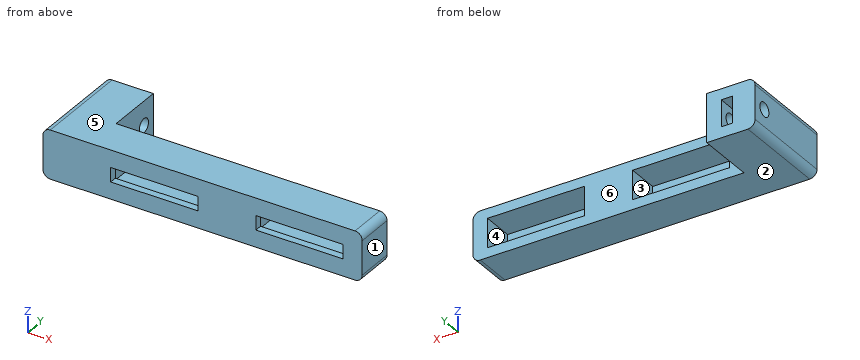
```python
from build123d import *

# Parameters (mm, degrees)
SALIENTE_EXTRUIR1_DEPTH = 10
REDONDEO5_R             = 1.5
CROQUIS3_W              = 20
CROQUIS3_H              = 6
CORTAR_EXTRUIR1_DEPTH   = 6.5
CROQUIS4_W              = 18
CROQUIS4_H              = 2.95
CORTAR_EXTRUIR2_DEPTH   = 1.5
CROQUIS5_R              = 1.45
CORTAR_EXTRUIR3_DEPTH   = 10
CROQUIS6_W              = 2.35
CROQUIS6_H              = 5.5
CORTAR_EXTRUIR4_DEPTH   = 6


with BuildPart() as part:
    # Croquis2 → Saliente-Extruir1 (new body)
    with BuildSketch(Plane.XY):
        Polygon((-160.336548935, 23.55779901), (-160.336548935, 3.55779901), (-94.336548935, 3.55779901), (-94.336548935, 11.55779901), (-150.336548935, 11.55779901), (-150.336548935, 23.55779901), align=None)
    extrude(amount=SALIENTE_EXTRUIR1_DEPTH)

    # Redondeo5
    redondeo5_edges = [part.edges().sort_by_distance(p)[0] for p in [
        (-94.336548935, 7.55779901, 10),
        (-94.336548935, 7.55779901, 0),
        (-160.336548935, 13.55779901, 10),
        (-160.336548935, 13.55779901, 0),
    ]]
    fillet(redondeo5_edges, radius=REDONDEO5_R)

    # Croquis3 → Cortar-Extruir1 (cut)
    with BuildSketch(Plane(origin=(0, 11.55779901, 0), x_dir=(1, 0, 0), z_dir=(0, 1, 0))):
        with Locations((-107.336548935, -5)):
            Rectangle(CROQUIS3_W, CROQUIS3_H)
        with Locations((-137.336548935, -5)):
            Rectangle(CROQUIS3_W, CROQUIS3_H)
    extrude(amount=-CORTAR_EXTRUIR1_DEPTH, mode=Mode.SUBTRACT)

    # Croquis4 → Cortar-Extruir2 (cut)
    with BuildSketch(Plane(origin=(0, 5.05779901, 0), x_dir=(1, 0, 0), z_dir=(0, 1, 0))):
        with Locations((-107.336548935, -4.975)):
            Rectangle(CROQUIS4_W, CROQUIS4_H)
        with Locations((-137.336548935, -4.975)):
            Rectangle(CROQUIS4_W, CROQUIS4_H)
    extrude(amount=-CORTAR_EXTRUIR2_DEPTH, mode=Mode.SUBTRACT)

    # Croquis5 → Cortar-Extruir3 (cut)
    with BuildSketch(Plane(origin=(-150.336548935, 0, 0), x_dir=(0, 0, -1), z_dir=(1, 0, 0))):
        with Locations((-5, 20.55779901)):
            Circle(CROQUIS5_R)
    extrude(amount=-CORTAR_EXTRUIR3_DEPTH, mode=Mode.SUBTRACT)

    # Croquis6 → Cortar-Extruir4 (cut)
    with BuildSketch(Plane(origin=(0, 23.55779901, 0), x_dir=(1, 0, 0), z_dir=(0, 1, 0))):
        with Locations((-154.511548935, -5)):
            Rectangle(CROQUIS6_W, CROQUIS6_H)
    extrude(amount=-CORTAR_EXTRUIR4_DEPTH, mode=Mode.SUBTRACT)


solid = part.part
```
CAD build for the part. Positions are in the model's coordinates, mm. Face numbers are marked on the shaded views. A direction names the side the tool comes from. Round coordinates to 2 decimals unless told otherwise and drop trailing zeros. Order: outer loops, then holes, each group sorted by start corner. A loop starts at its lowest first (then second) coordinate and runs counter-clockwise, first axis right, second up. Notation, with made-up numbers: (11.25, 11.5) - (69.25, 11.5) arc R35 cw to (69.25, 50.5) - close; hole circle Ø1 at (40, 3). An arc over 180 degrees is marked (long way). Answer as CSV lines item,"result". Start each with the question number.
1. Drill centre lines: L1, parallel to X at y = 10.5, z = 4.5; L2, parallel to Z at x = -134.5, y = 5.5; L3, parallel to Y at x = -152, z = 5. Where is each one in solid material? Low to high. Write a range as [from, to].
2. Saw through at A-A, the plane x = -115.5. Write the cut outline in (y, z), and give its area (3 significant figures).
3. Saw through at D-D, the plane y = 12.5. Write the cut outline in (x, z).
4. Saw through at C-C, the plane x = -154.5. Write the cut outline in (y, z).
5. Tool access for the marked faces 4, 5 and 6: list every direction of +Z, -Z, +X, -X, +Y, -Y with a clear straight run to the whole face (end or side of a thin tool).
6. Saw through at B-B, the plane z = 5. Count the separate pieces of the cut face and the enclosed holes in it, and give its area (3 significant figures).
7. Pin check, flat tips, straight feed: pin 1 (1 mm diameter, centred on y = 13.5, z = 5, fed in from +X); pin 2 (1.2 mm diameter, centred on x = -154.5, z = 4.5, fed in from +Y); pin 3 (1.7 mm diameter, centred on y = 20.56, z = 5, fed in from +X); pin 4 (5 mm diameter, centred on x = -111, z = 3.5, fed in from +Y). Stop position of each tip, or through.
8. Pull direction X, two halves, no side cores. Call the marked faces 1, 2 and 3: +X half, -X half, draft (parallel to the pull), parting line (faces both ways), or undercut.
Model answer:
1,L1,"x = [-160.34, -147.34], [-127.34, -117.34], [-97.34, -94.34]"
1,L2,"z = [0, 2], [8, 10]"
1,L3,"y = [3.56, 19.11], [22.01, 23.56]"
2,outline,"(3.56, 0) - (11.56, 0) - (11.56, 2) - (5.06, 2) - (5.06, 3.5) - (3.56, 3.5) - close; (3.56, 6.45) - (5.06, 6.45) - (5.06, 8) - (11.56, 8) - (11.56, 10) - (3.56, 10) - close"
2,area,"36.6 mm²"
3,outline,"(-160.34, 1.5) arc R1.5 ccw to (-158.84, 0) - (-150.34, 0) - (-150.34, 10) - (-158.84, 10) arc R1.5 ccw to (-160.34, 8.5) - close"
4,outline,"(3.56, 0) - (23.56, 0) - (23.56, 2.25) - (17.56, 2.25) - (17.56, 7.75) - (23.56, 7.75) - (23.56, 10) - (3.56, 10) - close"
5,face 4,"+Y"
5,face 5,"+Z, +X, -X, +Y, -Y"
5,face 6,"+Z, -Z, +X, +Y"
6,separate pieces,"5"
6,enclosed holes,"0"
6,area,"298 mm²"
7,pin 1,"stops at x = -150.34"
7,pin 2,"stops at y = 17.56"
7,pin 3,"passes through"
7,pin 4,"stops at y = 11.56"
8,face 1,"+X half"
8,face 2,"draft"
8,face 3,"undercut"
